Input: part model. Units: mm. Frame: model coordinates. Face numbers are marked on the shaded views. A direction names the side the tool comes from. Round coordinates to 2 decimals unless told otherwise and drop trailing zeros. Loops run counter-clockwise (first coordinate to the right, second up) from the corner with the lowest first, then second, coordinate; pieces in that order, holes last. Notation, with made-up numbers: M -29,87.25 L -8,87.25 A33 ccw -8,122.25 Z; hole C 30,60 d9. An arc over 180 degrees is marked long. Put each result on its own line as item: value. Start each with the question number.
1) Section D-D on y = 5. Output: boundary loops of the cut face in (x, z).
2) Section A-A on x = 12. Output: boundary loops of the cut face in (y, z), plus the area to 3 significant figures.
3) Reachability of the marked faces 5, 6, 7, 8 and 9 from +Z, -Z, +X, -X, +Y, -Y: full face, straight path, thin tool, end or side. Return the list, or none.
4) Draft query along X for the marked faces 1, 2, 3 and 4. Return one class per face: +X half, -X half, draft (parallel to the pull), parting line (faces both ways), or undercut.
5) Section B-B on y = 23. Output: boundary loops of the cut face in (x, z), plus the area to 3 significant figures.
6) Section C-C on z = 1.25. Output: boundary loops of the cut face in (x, y), plus the area to 3 significant figures.
7) Line query: probe 1 along X at (y, z) = (12.25, 5.75); probe 2 along Z at (x, y) = (16.75, 15); probe 3 along Y at (x, z) = (12, 3.65). Output: solid intervals per line, ascending.
8) Pin query (flat end, axial travel): pin 1 (5.5 mm diameter, centred on y = 16.5, z = 5.5, fed in from +X); pin 2 (2 mm diameter, centred on y = 16.5, z = 9, fed in from +X); pin 3 (3 mm diameter, centred on y = 21, z = 9, fed in from -X); pin 4 (11 mm diameter, centred on x = 37.5, y = 18, fed in from +Z). Return the tip coordinate at first contact, or that it passes through.
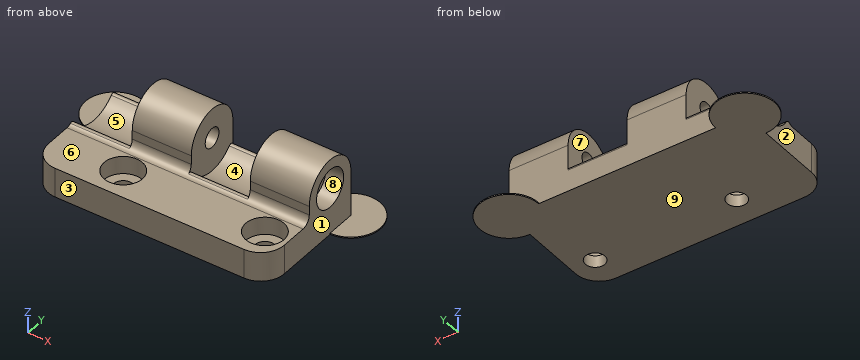
from build123d import *

# Parameters (mm, degrees)
F1_DEPTH       = 5
F3_D           = 3.3
F3_CBORE_D     = 6.5
F3_CBORE_DEPTH = 3
F5_DEPTH       = 40
F6_R           = 1.5
F8_D           = 3.3
F8_CBORE_D     = 6.5
F8_CBORE_DEPTH = 3
F10_R          = 5.75
F11_DEPTH      = 10
F13_R          = 5.75
F14_DEPTH      = 10.001
F15_R          = 0.5
F16_R          = 5
F17_DEPTH      = 0.2


with BuildPart() as f1:
    # F0 (on Top) → F1 (new body)
    with BuildSketch(Plane.XY):
        with BuildLine():
            ThreePointArc((0, 4), (1.1715728753, 1.1715728753), (4, 0))
            Line((4, 0), (36, 0))
            ThreePointArc((36, 0), (38.8284271247, 1.1715728753), (40, 4))
            Line((40, 4), (40, 14))
            Line((40, 14), (0, 14))
            Line((0, 14), (0, 4))
        make_face()
    extrude(amount=F1_DEPTH)

    # F3 (through all)
    with Locations(Plane.XY.offset(5)):
        with Locations((12, 5), (36, 5)):
            CounterBoreHole(F3_D / 2, F3_CBORE_D / 2, F3_CBORE_DEPTH)

    # F4 (on Right) → F5 (join)
    with BuildSketch(Plane.YZ):
        with BuildLine():
            Line((10, 8), (10, 0))
            Line((10, 0), (20, 0))
            Line((20, 0), (20, 8))
            ThreePointArc((20, 8), (15, 13), (10, 8))
        make_face()
    extrude(amount=F5_DEPTH)

    # F6
    f6_edges = [f1.edges().sort_by_distance(p)[0] for p in [
        (20, 10, 5),
    ]]
    fillet(f6_edges, radius=F6_R)

    # F8 (through all)
    with Locations(Plane.YZ.offset(40)):
        with Locations((15, 8)):
            CounterBoreHole(F8_D / 2, F8_CBORE_D / 2, F8_CBORE_DEPTH)

    # F10 (on offset) → F11 (cut)
    with BuildSketch(Plane.YZ.offset(30)):
        with Locations((15, 8)):
            Circle(F10_R)
    extrude(amount=-F11_DEPTH, mode=Mode.SUBTRACT)

    # F13 (on offset) → F14 (cut, through all)
    with BuildSketch(Plane.YZ.offset(10)):
        with Locations((15, 8)):
            Circle(F13_R)
    extrude(amount=-F14_DEPTH, mode=Mode.SUBTRACT)

    # F15
    f15_edges = [f1.edges().sort_by_distance(p)[0] for p in [
        (5, 9.745712, 5.664415),
        (5, 20, 5.160546),
        (25, 20, 5.160546),
        (25, 9.745712, 5.664415),
    ]]
    fillet(f15_edges, radius=F15_R)

    # F16 (on Top) → F17 (join)
    with BuildSketch(Plane.XY):
        with Locations((0, 20)):
            Circle(F16_R)
        with Locations((40, 20)):
            Circle(F16_R)
    extrude(amount=F17_DEPTH)


solid = f1.part
Geometry results:
1. outline: M 0,0 L 10.35,0 L 10.35,2 L 8.75,2 L 8.75,5 L 0,5 Z; M 13.65,0 L 34.35,0 L 34.35,2 L 32.75,2 L 32.75,5 L 15.25,5 L 15.25,2 L 13.65,2 Z; M 37.65,0 L 40,0 L 40,5 L 39.25,5 L 39.25,2 L 37.65,2 Z
2. outline: M 0,0 L 3.35,0 L 3.35,2 L 1.75,2 L 1.75,5 L 0,5 Z; M 6.65,0 L 20,0 L 20,8 A5 ccw 10,8 L 10,6.5 A1.5 cw 8.5,5 L 8.25,5 L 8.25,2 L 6.65,2 Z; hole C 15,8 d3.3
2. area: 135 mm²
3. face 5: +Z, -X
3. face 6: +Z, +X, -X, -Y
3. face 7: +Z
3. face 8: +X
3. face 9: -Z, +X, -X, +Y, -Y
4. face 1: +X half
4. face 2: -X half
4. face 3: draft
4. face 4: undercut
5. outline: M -4,0 L 4,0 L 4,0.2 L -4,0.2 Z; M 36,0 L 44,0 L 44,0.2 L 36,0.2 Z
5. area: 3.20 mm²
6. outline: M 0,4 A4 ccw 4,0 L 36,0 A4 ccw 40,4 L 40,20 L 0,20 Z; hole C 12,5 d3.3; hole C 36,5 d3.3
6. area: 776 mm²
7. probe 1: x = 10 to 20, 30 to 40
7. probe 2: z = 0 to 6.35, 9.65 to 13
7. probe 3: y = 0 to 1.75, 8.25 to 20
8. pin 1: stops at x = 40
8. pin 2: stops at x = 37
8. pin 3: stops at x = 10
8. pin 4: stops at z = 13
